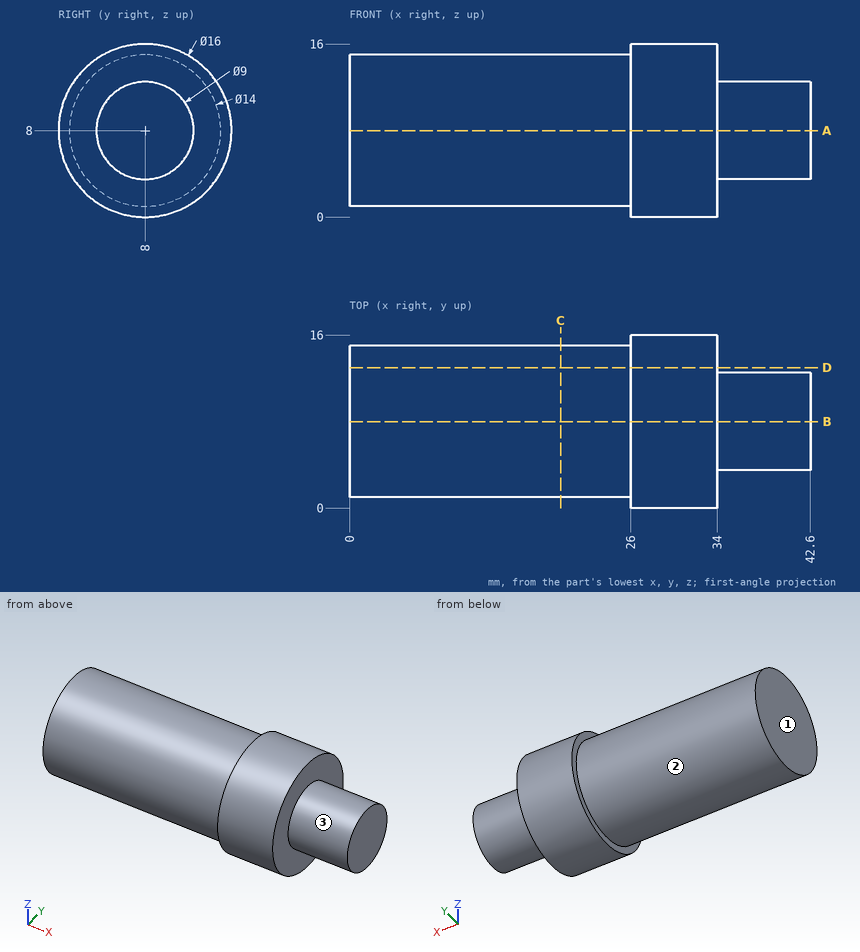
Source: three-view drawing plus pictorial views. Frame: mm from the lowest corner of the part. A direction names the side the tool comes from. Coordinates: 2 decimals unless noted, no trailing zeros. Loops run counter-clockwise (first coordinate to the right, second up) from the corner with the lowest first, then second, coordinate; pieces in that order, holes last. Notation, with made-up numbers: (14, 38.25) - (35, 38.25) arc R27 ccw to (35, 68.25) - close; hole circle Ø9 at (-38.75, 12). An arc over 180 degrees is marked (long way). Answer in a Markdown table with one row per item. Add a question column.
Item 1: Contact query for flat-ended pins moving along their axis: P1, Ø1, axis at x = 14, z = 7, coming from the +Y side; P2, Ø4, axis at x = 27, y = 14, coming from the -Z side; P3, Ø5, axis at y = 13.5, z = 3.5, coming from the +X side. Output: stop coordinate, or through.
Item 2: Section query A-A on z = 8. Return the cut outline in (x, y).
Item 3: Access query for the marked faces 1, 2 and 3. Directions: +Z, -Z, +X, -X, +Y, -Y. A direction counts if a zero-diameter tool reaches every point of the face in a straight line with its end or side. Return the directions, or none.
Item 4: Section query D-D on y = 13. Return the cut outline in (x, z) (3 decimals).
Item 5: Line query: line 1 along X through (y, z) = (0.5, 10.25); line 2 along Y through (x, z) = (30, 8.25); line 3 along Z through (x, y) = (19, 8). Output: solid intervals per line, ascending. Write a range as [from, to].
Item 6: Section query C-C on x = 19.5. Return the cut outline in (y, z), then the cut area to 3 significant figures.
Recorded:
| question | item | result |
|---|---|---|
| 1 | P1 | y = 14.98 |
| 1 | P2 | z = 1.07 |
| 1 | P3 | x = 34 |
| 2 | outline | (0, 1) - (26, 1) - (26, 0) - (34, 0) - (34, 3.5) - (42.6, 3.5) - (42.6, 12.5) - (34, 12.5) - (34, 16) - (26, 16) - (26, 15) - (0, 15) - close |
| 3 | face 1 | +Z, -Z, -X, +Y, -Y |
| 3 | face 2 | -X |
| 3 | face 3 | +X |
| 4 | outline | (0, 3.101) - (26, 3.101) - (26, 1.755) - (34, 1.755) - (34, 14.245) - (26, 14.245) - (26, 12.899) - (0, 12.899) - close |
| 5 | line 1 | [26, 34] |
| 5 | line 2 | [0, 16] |
| 5 | line 3 | [1, 15] |
| 6 | outline | circle Ø14 at (8, 8) |
| 6 | area | 154 mm^2 |
